from build123d import *

# Parameters (mm, degrees)
SKETCH_R        = 4
PAD_DEPTH       = 10
SKETCH001_R     = 2.25
PAD001_DEPTH    = 2.25
SKETCH002_R     = 3.5
PAD002_DEPTH    = 1.5
CHAMFER_SIZE    = 0.5
SKETCH003_R     = 1.6
POCKET_DEPTH    = 8
CHAMFER001_SIZE = 0.3
CHAMFER002_SIZE = 0.4


with BuildPart() as part:
    # Sketch → Pad (new body)
    with BuildSketch(Plane.XZ):
        Circle(SKETCH_R)
    extrude(amount=PAD_DEPTH)

    # Sketch001 → Pad001 (join)
    with BuildSketch(Plane.XZ):
        Circle(SKETCH001_R)
    extrude(amount=-PAD001_DEPTH)

    # Sketch002 (on Face5 of Pad001) → Pad002 (join)
    with BuildSketch(Plane(origin=(0, 2.25, 0), x_dir=(1, 0, 0), z_dir=(0, 1, 0))):
        Circle(SKETCH002_R)
    extrude(amount=PAD002_DEPTH)

    # Chamfer
    chamfer_edges = [part.edges().sort_by_distance(p)[0] for p in [
        (-3.5, 3.75, 0),
        (-3.5, 2.25, 0),
        (-4, 0, 0),
    ]]
    chamfer(chamfer_edges, length=CHAMFER_SIZE)

    # Sketch003 (on Face3 of Chamfer) → Pocket (cut)
    with BuildSketch(Plane.XZ.offset(10)):
        Circle(SKETCH003_R)
    extrude(amount=-POCKET_DEPTH, mode=Mode.SUBTRACT)

    # Chamfer001
    chamfer001_edges = [part.edges().sort_by_distance(p)[0] for p in [
        (-4, -10, 0),
        (-1.6, -10, 0),
    ]]
    chamfer(chamfer001_edges, length=CHAMFER001_SIZE)

    # Chamfer002
    chamfer002_edges = [part.edges().sort_by_distance(p)[0] for p in [
        (-1.6, -2, 0),
    ]]
    chamfer(chamfer002_edges, length=CHAMFER002_SIZE)


solid = part.part
Work out the finished part from the listing and answer in its coordinate system (mm). A direction names the side the tool comes from. Give positions to 0.01 mm unless a question says otherwise; leave off trailing zeros. Loops run counter-clockwise (first coordinate to the right, second up) from the corner with the lowest first, then second, coordinate; pieces in that order, holes last. Notation, with made-up numbers: (-13, 31.5) - (12, 31.5) arc R9 cw to (12, 39.5) - close; hole circle Ø2 at (81.25, -37). An arc over 180 degrees is marked (long way). Answer in a Markdown table with one row per item.
(1) Section A-A (x = 0) is taken. Give the vertices of the cut face in (y, z), and give its area (3 significant figures).
Results list:
| item | result |
|---|---|
| outline | (-10, -3.7) - (-9.7, -4) - (-0.5, -4) - (0, -3.5) - (0, -2.25) - (2.25, -2.25) - (2.25, -3) - (2.75, -3.5) - (3.25, -3.5) - (3.75, -3) - (3.75, 3) - (3.25, 3.5) - (2.75, 3.5) - (2.25, 3) - (2.25, 2.25) - (0, 2.25) - (0, 3.5) - (-0.5, 4) - (-9.7, 4) - (-10, 3.7) - (-10, 1.9) - (-9.7, 1.6) - (-2.4, 1.6) - (-2, 1.2) - (-2, -1.2) - (-2.4, -1.6) - (-9.7, -1.6) - (-10, -1.9) - close |
| area | 74.3 mm² |
(2) Consider L1, parallel to Z at x = 0, y = -7.5; L2, parallel to Y at x = 1.75, z = 2; L3, parallel to Y at x = -0.5, z = -0.5. Determine where each line is inside the solid, lowest interval first. Write a range as [from, to].
Results list:
| item | result |
|---|---|
| L1 | z = [-4, -1.6], [1.6, 4] |
| L2 | y = [-10, 0], [2.25, 3.75] |
| L3 | y = [-2, 3.75] |
(3) Section C-C (y = -5.75) is taken. Give the vertices of the cut face in (x, z).
Results list:
| item | result |
|---|---|
| outline | circle Ø8 at (0, 0); hole circle Ø3.2 at (0, 0) |
(4) For a pull along Y with two mould halves and no side action, classify faces 1 (the face through (-2, -10, 1)), 2 (the face through (3.233, 2.996, 1.341)), 3 (the face through (-0.29, 1.11, 2.23)), 4 (the face through (0.7, 0, -2.3)) as pulls with the +Y half, pulls with the -Y half, needs draft (parallel to the pull), parting line crosses it, or undercut.
Results list:
| item | result |
|---|---|
| face 1 | pulls with the -Y half |
| face 2 | needs draft |
| face 3 | undercut |
| face 4 | undercut |
(5) Section B-B (z = 0) is taken. Give the vertices of the cut face in (x, y), and give its area (3 significant figures).
Results list:
| item | result |
|---|---|
| outline | (-4, -9.7) - (-3.7, -10) - (-1.9, -10) - (-1.6, -9.7) - (-1.6, -2.4) - (-1.2, -2) - (1.2, -2) - (1.6, -2.4) - (1.6, -9.7) - (1.9, -10) - (3.7, -10) - (4, -9.7) - (4, -0.5) - (3.5, 0) - (2.25, 0) - (2.25, 2.25) - (3, 2.25) - (3.5, 2.75) - (3.5, 3.25) - (3, 3.75) - (-3, 3.75) - (-3.5, 3.25) - (-3.5, 2.75) - (-3, 2.25) - (-2.25, 2.25) - (-2.25, 0) - (-3.5, 0) - (-4, -0.5) - close |
| area | 74.3 mm² |
(6) Flat-ended cylindrical pins translate along their axes: pin 1 Ø2 at (y, z) = (-1, 2) entering from +X; pin 2 Ø4 at (x, z) = (0, 0) entering from -Y; pin 3 Ø1.9 at (x, z) = (-0.5, -0.5) entering from -Y; pin 4 Ø2 at (y, z) = (-5.5, 3) entering from +X. Find the tip coordinate at first contact, or state that the pin passes through.
Results list:
| item | result |
|---|---|
| pin 1 | stops at x = 3.87 |
| pin 2 | stops at y = -10 |
| pin 3 | stops at y = -9.76 |
| pin 4 | stops at x = 3.46 |
(7) A tool of negligible diameter and unlimited length cuts with its end or side. For faces 5 (the face through (-1.27, -6.1, -0.97)), 6 (the face through (0, 3.75, 0)), from which of +Z, -Z, +X, -X, +Y, -Y can it reach the whole face along a straight path? Write none if from no direction.
Results list:
| item | result |
|---|---|
| face 5 | -Y |
| face 6 | +Z, -Z, +X, -X, +Y |
